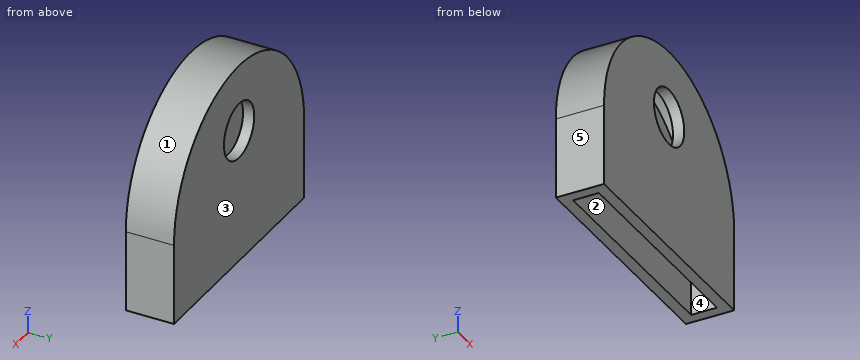
from build123d import *

# Parameters (mm, degrees)
F0_W     = 21.5
F0_H     = 7.25
F1_DEPTH = 1
F3_DEPTH = 2.3
F5_DEPTH = 1
F6_R     = 2.5
F7_DEPTH = 4.301


with BuildPart() as f1:
    # F0 (on Front) → F1 (new body)
    with BuildSketch(Plane.XZ):
        with Locations((10.75, 3.625)):
            Rectangle(F0_W, F0_H)
        with BuildLine():
            ThreePointArc((21.5, 7.25), (10.75, 18), (0, 7.25))
            Line((0, 7.25), (21.5, 7.25))
        make_face()
    extrude(amount=F1_DEPTH)

    # F2 (on face) → F3 (join)
    with BuildSketch(Plane.XZ.offset(1)):
        with BuildLine():
            Line((20.5, 7.25), (20.5, 0))
            Line((20.5, 0), (21.5, 0))
            Line((21.5, 0), (21.5, 7.25))
            ThreePointArc((21.5, 7.25), (10.75, 18), (0, 7.25))
            Line((0, 7.25), (0, 0))
            Line((0, 0), (1, 0))
            Line((1, 0), (1, 7.25))
            ThreePointArc((1, 7.25), (10.75, 17), (20.5, 7.25))
        make_face()
    extrude(amount=F3_DEPTH)

    # F4 (on face) → F5 (join)
    with BuildSketch(Plane.XZ.offset(3.3)):
        with BuildLine():
            Line((0, 7.25), (0, 0))
            Line((0, 0), (21.5, 0))
            Line((21.5, 0), (21.5, 7.25))
            ThreePointArc((21.5, 7.25), (10.75, 18), (0, 7.25))
        make_face()
    extrude(amount=F5_DEPTH)

    # F6 (on face) → F7 (cut, through all)
    with BuildSketch(Plane.XZ.offset(4.3)):
        with Locations((10.75, 12)):
            Circle(F6_R)
    extrude(amount=-F7_DEPTH, mode=Mode.SUBTRACT)


solid = f1.part
Could you check a few things on this model? Use its own coordinates, in mm. Face numbers are marked on the shaded views. A direction names the side the tool comes from. Coordinates: 2 decimals unless noted, no trailing zeros. Loops run counter-clockwise (first coordinate to the right, second up) from the corner with the lowest first, then second, coordinate; pieces in that order, holes last. Notation, with made-up numbers: (66.5, 13) -> (79.5, 13) arc R26 ccw to (79.5, 48) -> close; hole circle Ø10 at (-26, -23). An arc over 180 degrees is marked (long way). Answer in a Markdown table with one row per item.
(1) Thinking about a two-plate mould opening in Y: for the marked faces 1, 2 and 3, which applies, released by +Y, released by -Y, zero draft, split by the parting line, or undercut?
Results found:
| item | result |
|---|---|
| face 1 | zero draft |
| face 2 | undercut |
| face 3 | released by +Y |
(2) For the marked faces 4 and 5, which set-ups out of +Z, -Z, +X, -X, +Y, -Y let a thin tool reach every point of the face, with its end or its side?
Results found:
| item | result |
|---|---|
| face 4 | -Z |
| face 5 | +Z, -Z, -X, +Y, -Y |
(3) Imagine slicing it at A-A (x = 10.75). List the corners of the cut face in (y, z) for me.
Results found:
| item | result |
|---|---|
| outline | (-4.3, 0) -> (-3.3, 0) -> (-3.3, 9.5) -> (-4.3, 9.5) -> close; (-4.3, 14.5) -> (-3.3, 14.5) -> (-3.3, 17) -> (-1, 17) -> (-1, 14.5) -> (0, 14.5) -> (0, 18) -> (-4.3, 18) -> close; (-1, 0) -> (0, 0) -> (0, 9.5) -> (-1, 9.5) -> close |
(4) If I drill on probe 1 along Z at (x, y) = (10.75, -0.5); probe 2 along Y at (x, z) = (18.5, 11.25); probe 3 along X at (y, z) = (-2.15, 7.25), over which ranges is the centre line in solid material (lowest first)?
Results found:
| item | result |
|---|---|
| probe 1 | z = 0 to 9.5, 14.5 to 18 |
| probe 2 | y = -4.3 to -3.3, -1 to 0 |
| probe 3 | x = 0 to 1, 20.5 to 21.5 |
(5) Imagine slicing it at B-B (z = 4.25). List the corners of the cut face in (x, y) for me, plus the area to 3 significant figures.
Results found:
| item | result |
|---|---|
| outline | (0, -4.3) -> (21.5, -4.3) -> (21.5, 0) -> (0, 0) -> close; hole (1, -3.3) -> (20.5, -3.3) -> (20.5, -1) -> (1, -1) -> close |
| area | 47.6 mm^2 |
(6) Imagine slicing it at C-C (z = 12.75). List the corners of the cut face in (x, y) for me.
Results found:
| item | result |
|---|---|
| outline | (1.51, -4.3) -> (8.37, -4.3) -> (8.37, -3.3) -> (2.7, -3.3) -> (2.7, -1) -> (8.37, -1) -> (8.37, 0) -> (1.51, 0) -> close; (13.13, -4.3) -> (19.99, -4.3) -> (19.99, 0) -> (13.13, 0) -> (13.13, -1) -> (18.8, -1) -> (18.8, -3.3) -> (13.13, -3.3) -> close |
(7) Imagine slicing it at D-D (y = -0.3). List the corners of the cut face in (x, z) for me.
Results found:
| item | result |
|---|---|
| outline | (0, 0) -> (21.5, 0) -> (21.5, 7.25) arc R10.75 ccw to (0, 7.25) -> close; hole circle Ø5 at (10.75, 12) |
(8) Will these pins go through, and if not, where does the flat tip stop? pin 1 Ø8.5 at (x, z) = (9, 10.5) entering from +Y; pin 2 Ø1.5 at (y, z) = (-2, 11.5) entering from -X; pin 3 Ø1.5 at (x, z) = (2, 15.5) entering from +Y.
Results found:
| item | result |
|---|---|
| pin 1 | stops at y = 0 |
| pin 2 | stops at x = 0.59 |
| pin 3 | passes through |
